Source: CAD feature listing. Evaluate the final solid. Frame: model axes, mm. Round coordinates to 2 decimals unless told otherwise and drop trailing zeros. Write each loop counter-clockwise with the first axis right and the second up, starting at its lowest first coordinate (ties: lowest second). Pieces come first, ordered by that corner, then holes.
from build123d import *

# Parameters (mm, degrees)
RESSALTO_EXTRUS_O2_DEPTH           = 2
RESSALTO_EXTRUS_O2_OTHER_WAY_DEPTH = 2
RESSALTO_EXTRUS_O2_OTHER_WAY_TAPER = 10


with BuildPart() as part:
    # Esboço6 → Ressalto-extrusão2 (new body)
    with BuildSketch(Plane.XY):
        with BuildLine():
            ThreePointArc((-10, 0), (-2.928932188, 2.928932188), (0, 10))
            Line((0, 10), (0, 33))
            ThreePointArc((0, 33), (-2.928932188, 40.071067812), (-10, 43))
            Line((-10, 43), (-36.5, 43))
            ThreePointArc((-36.5, 43), (-43.571067812, 40.071067812), (-46.5, 33))
            Line((-46.5, 33), (-46.5, 10))
            ThreePointArc((-46.5, 10), (-43.571067812, 2.928932188), (-36.5, 0))
            Line((-36.5, 0), (-10, 0))
        make_face()
    extrude(amount=-RESSALTO_EXTRUS_O2_DEPTH)

    # Esboço6 → Ressalto-extrusão2 other way (add)
    with BuildSketch(Plane.XY):
        with BuildLine():
            ThreePointArc((-10, 0), (-2.928932188, 2.928932188), (0, 10))
            Line((0, 10), (0, 33))
            ThreePointArc((0, 33), (-2.928932188, 40.071067812), (-10, 43))
            Line((-10, 43), (-36.5, 43))
            ThreePointArc((-36.5, 43), (-43.571067812, 40.071067812), (-46.5, 33))
            Line((-46.5, 33), (-46.5, 10))
            ThreePointArc((-46.5, 10), (-43.571067812, 2.928932188), (-36.5, 0))
            Line((-36.5, 0), (-10, 0))
        make_face()
    extrude(amount=RESSALTO_EXTRUS_O2_OTHER_WAY_DEPTH, taper=RESSALTO_EXTRUS_O2_OTHER_WAY_TAPER)


solid = part.part
1) Contact query for flat-ended pins moving along their axis: P1, Ø1.5, axis at x = -35, z = 1, coming from the +Y side; P2, Ø1.5, axis at x = -7.5, z = 0, coming from the -Y side. Output: stop coordinate, or through.
Taken from the geometry:
P1: stops at y = 42.96
P2: stops at y = 0.15
2) Material intervals for line 1 (Y direction, x = -37, z = -1.2); line 2 (X direction, y = 5.5, z = 1.35); line 3 (X direction, y = 34, z = -0.7), sorted ascending.
Taken from the geometry:
line 1: y = 0.01 to 42.99
line 2: x = -45.16 to -1.34
line 3: x = -46.45 to -0.05
3) Section query A-A on z = -0.6. Return the cut outline in (x, y), then the cut area to 3 significant figures.
Taken from the geometry:
outline: (-46.5, 10) arc R10 ccw to (-36.5, 0) - (-10, 0) arc R10 ccw to (0, 10) - (0, 33) arc R10 ccw to (-10, 43) - (-36.5, 43) arc R10 ccw to (-46.5, 33) - close
area: 1,910 mm2
